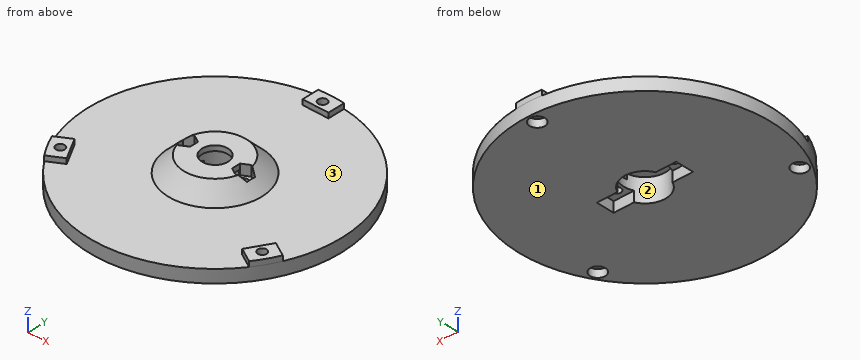
from build123d import *

# Parameters (mm, degrees)
SKETCH001_W        = 30.6
SKETCH001_H        = 7
POCKET_DEPTH       = 4
SKETCH002_R        = 1.7
POCKET001_DEPTH    = 7.001
POCKET002_DEPTH    = 4
PAD_DEPTH          = 2
SKETCH005_R        = 1.7
POCKET003_DEPTH    = 283.930739
SKETCH006_R        = 2.95
POCKET004_DEPTH    = 3
POLARPATTERN_COUNT = 3


with BuildPart() as part:
    # Sketch → Revolution (revolve)
    with BuildSketch(Plane.XZ):
        Polygon((5, 11), (5, 9), (8.2, 9), (8.2, 0), (48.8, 0), (48.8, 5), (18, 5), (12, 11), align=None)
    revolve(axis=Axis((0, 0, 0), (0, 0, 1)))

    # Sketch001 (on Face4 of Revolution) → Pocket (cut)
    with BuildSketch(Plane(origin=(0, 0, 0), x_dir=(1, 0, 0), z_dir=(0, 0, -1))):
        Rectangle(SKETCH001_W, SKETCH001_H)
    extrude(amount=-POCKET_DEPTH, mode=Mode.SUBTRACT)

    # Sketch002 (on Face11 of Pocket) → Pocket001 (cut, through all)
    with BuildSketch(Plane(origin=(0, 0, 4), x_dir=(1, 0, 0), z_dir=(0, 0, -1))):
        with Locations((-11, 0)):
            Circle(SKETCH002_R)
        with Locations((11, 0)):
            Circle(SKETCH002_R)
    extrude(amount=-POCKET001_DEPTH, mode=Mode.SUBTRACT)

    # Sketch003 (on Face2 of Pocket001) → Pocket002 (cut)
    with BuildSketch(Plane(origin=(0, 0, 11), x_dir=(-1, 0, 0), z_dir=(0, 0, 1))):
        Polygon((-11, -3.35), (-8.098815, -1.675), (-8.098815, 1.675), (-11, 3.35), (-13.901185, 1.675), (-13.901185, -1.675), align=None)
        Polygon((11, -3.35), (13.901185, -1.675), (13.901185, 1.675), (11, 3.35), (8.098815, 1.675), (8.098815, -1.675), align=None)
    extrude(amount=-POCKET002_DEPTH, mode=Mode.SUBTRACT)

    # Sketch004 (on Face18 of Pocket002) → Pad (join)
    with BuildSketch(Plane(origin=(0, 0, 5), x_dir=(-1, 0, 0), z_dir=(0, 0, 1))):
        with BuildLine():
            ThreePointArc((-5, -48.543177), (0, -48.8), (5, -48.543177))
            Line((5, -42), (5, -48.543177))
            Line((-5, -42), (5, -42))
            Line((-5, -48.543177), (-5, -42))
        make_face()
    pad = extrude(amount=PAD_DEPTH)

    # Sketch005 (on Face35 of Pad) → Pocket003 (cut, through all)
    with BuildSketch(Plane(origin=(0, 0, 7), x_dir=(-1, 0, 0), z_dir=(0, 0, 1))):
        with Locations((0, -45)):
            Circle(SKETCH005_R)
    pocket003 = extrude(amount=-POCKET003_DEPTH, mode=Mode.SUBTRACT)

    # Sketch006 (on Face23 of Pocket003) → Pocket004 (cut)
    with BuildSketch(Plane(origin=(0, 0, 0), x_dir=(1, 0, 0), z_dir=(0, 0, -1))):
        with Locations((0, -45)):
            Circle(SKETCH006_R)
    pocket004 = extrude(amount=-POCKET004_DEPTH, mode=Mode.SUBTRACT)

    # PolarPattern: Pad, Pocket003, Pocket004 ×3 about axis
    polarpattern_axis = Axis((0, 0, 5), (0, 0, 1))
    for i in range(1, POLARPATTERN_COUNT):
        add(pad.rotate(polarpattern_axis, i * 360 / POLARPATTERN_COUNT))
        add(pocket003.rotate(polarpattern_axis, i * 360 / POLARPATTERN_COUNT), mode=Mode.SUBTRACT)
        add(pocket004.rotate(polarpattern_axis, i * 360 / POLARPATTERN_COUNT), mode=Mode.SUBTRACT)


solid = part.part
Geometry: final body of the model. Coordinates: model frame, mm. Face numbers are marked on the shaded views. A direction names the side the tool comes from. Round coordinates to 2 decimals unless told otherwise and drop trailing zeros. Loops run counter-clockwise (first coordinate to the right, second up) from the corner with the lowest first, then second, coordinate; pieces in that order, holes last. Notation, with made-up numbers: M 13.25,-21 L 50.25,-21 A20 cw 50.25,11 Z; hole C -27,43 d8. An arc over 180 degrees is marked long. Put each result on its own line as item: value. Start each with the question number.
(1) Material intervals for line 1 along Y through (x, z) = (0, 4.65); line 2 along X through (y, z) = (45, 5.45); line 3 along Y through (x, z) = (25, 3.5), sorted ascending. Write a range as [from, to].
(2) Section query B-B (y = -22.5). Return loops of the section in (x, z).
(3) Section query C-C (y = 45). Return loops of the section in (x, z), then the cut area to 3 significant figures.
(4) Set-up query: the marked faces 1, 2 and 3. Return all of +Z, -Z, +X, -X, +Y, -Y with unobstructed straight access to the full face (end or side cutting, diameter ignored); none if empty.
(5) Contact query for flat-ended pins moving along their axis: pin 1 Ø3 at (y, z) = (0.5, 2) entering from +X; pin 2 Ø2.5 at (x, y) = (-11, 0) entering from +Z; pin 3 Ø3 at (x, y) = (37, -23.5) entering from +Z; pin 4 Ø2.5 at (y, z) = (0.5, 9) entering from +X. Output: stop coordinate, or through.
(6) Section query A-A (x = 0). Return loops of the section in (y, z).
(7) Section query D-D (x = 24.5). Return loops of the section in (y, z), then the cut area to 3 significant figures.
Findings below:
1. line 1: y = [-48.8, -8.2], [8.2, 43.3], [46.7, 48.8]
1. line 2: x = [-5, -1.7], [1.7, 5]
1. line 3: y = [-41.91, 41.91]
2. outline: M -43.3,0 L -41.92,0 L -41.92,3 L -40.67,3 L -40.67,7 L -43.3,7 Z; M -37.27,3 L -36.02,3 L -36.02,0 L 36.02,0 L 36.02,3 L 37.27,3 L 37.27,7 L 35.51,7 L 35.51,5 L -35.51,5 L -35.51,7 L -37.27,7 Z; M 40.67,3 L 41.92,3 L 41.92,0 L 43.3,0 L 43.3,7 L 40.67,7 Z
3. outline: M -18.88,0 L -2.95,0 L -2.95,3 L -1.7,3 L -1.7,7 L -5,7 L -5,5 L -18.88,5 Z; M 1.7,3 L 2.95,3 L 2.95,0 L 18.88,0 L 18.88,5 L 5,5 L 5,7 L 1.7,7 Z
3. area: 177 mm2
4. face 1: -Z, +X, -X, +Y, -Y
4. face 2: -Z
4. face 3: +Z
5. pin 1: stops at x = 48.8
5. pin 2: passes through
5. pin 3: stops at z = 7
5. pin 4: stops at x = 15.24
6. outline: M -48.8,0 L -8.2,0 L -8.2,9 L -5,9 L -5,11 L -12,11 L -18,5 L -48.8,5 Z; M 5,9 L 8.2,9 L 8.2,0 L 42.05,0 L 42.05,3 L 43.3,3 L 43.3,7 L 42,7 L 42,5 L 18,5 L 12,11 L 5,11 Z; M 46.7,3 L 47.95,3 L 47.95,0 L 48.8,0 L 48.8,7 L 46.7,7 Z
7. outline: M -42.2,0 L 42.2,0 L 42.2,5 L -42.2,5 Z
7. area: 422 mm2
